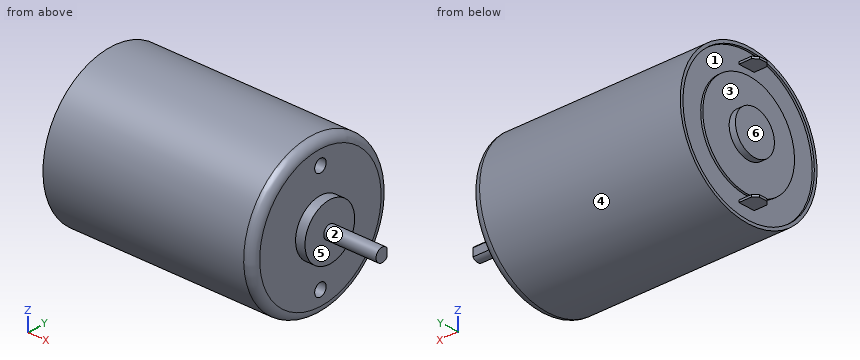
```python
from build123d import *

# Parameters (mm, degrees)
SKETCH1_R           = 17.9
MOTOR_BODY_DEPTH    = 25
SKETCH2_R           = 17.2
CUT_EXTRUDE1_DEPTH  = 0.5
SKETCH3_R           = 12
BOSS_EXTRUDE2_DEPTH = 0.5
SKETCH4_R           = 5.1
BOSS_EXTRUDE3_DEPTH = 1.5
FILLET1_R           = 2
SKETCH5_W           = 0.5
SKETCH5_H           = 4
BOSS_EXTRUDE4_DEPTH = 4
CHAMFER1_SIZE       = 1
SKETCH6_R           = 1.5
MOUNT_HOLES_DEPTH   = 6
SKETCH7_R           = 6.5
BOSS_EXTRUDE5_DEPTH = 2.25
SKETCH8_R           = 1.585
OUTPUT_SHAFT_DEPTH  = 12.5
CUT_EXTRUDE3_DEPTH  = 10


with BuildPart() as part:
    # Sketch1 → Motor-Body (new body, symmetric)
    with BuildSketch(Plane(origin=(0, 0, 0), x_dir=(0, 0, -1), z_dir=(1, 0, 0))):
        Circle(SKETCH1_R)
    extrude(amount=MOTOR_BODY_DEPTH, both=True)

    # Sketch2 → Cut-Extrude1 (cut)
    with BuildSketch(Plane.ZY.offset(25)):
        Circle(SKETCH2_R)
    extrude(amount=-CUT_EXTRUDE1_DEPTH, mode=Mode.SUBTRACT)

    # Sketch3 → Boss-Extrude2 (add, symmetric)
    with BuildSketch(Plane.ZY.offset(24.5)):
        Circle(SKETCH3_R)
    extrude(amount=BOSS_EXTRUDE2_DEPTH, both=True)

    # Sketch4 → Boss-Extrude3 (add, symmetric)
    with BuildSketch(Plane.ZY.offset(25)):
        Circle(SKETCH4_R)
    extrude(amount=BOSS_EXTRUDE3_DEPTH, both=True)

    # Fillet1
    fillet1_edges = [part.edges().sort_by_distance(p)[0] for p in [
        (25, 0, 17.9),
    ]]
    fillet(fillet1_edges, radius=FILLET1_R)

    # Sketch5 → Boss-Extrude4 (add)
    with BuildSketch(Plane.ZY.offset(24.5)):
        with Locations((-13.95, 0)):
            Rectangle(SKETCH5_W, SKETCH5_H)
        with Locations((13.95, 0)):
            Rectangle(SKETCH5_W, SKETCH5_H)
    extrude(amount=BOSS_EXTRUDE4_DEPTH)

    # Chamfer1
    chamfer1_edges = [part.edges().sort_by_distance(p)[0] for p in [
        (-28.5, 2, -13.95),
        (-28.5, -2, -13.95),
        (-28.5, 2, 13.95),
        (-28.5, -2, 13.95),
    ]]
    chamfer(chamfer1_edges, length=CHAMFER1_SIZE)

    # Sketch6 → Mount-Holes (cut)
    with BuildSketch(Plane(origin=(25, 0, 0), x_dir=(0, 0, -1), z_dir=(1, 0, 0))):
        with Locations((-12.5, 0)):
            Circle(SKETCH6_R)
        with Locations((12.5, 0)):
            Circle(SKETCH6_R)
    extrude(amount=-MOUNT_HOLES_DEPTH, mode=Mode.SUBTRACT)

    # Sketch7 → Boss-Extrude5 (add, symmetric)
    with BuildSketch(Plane(origin=(25, 0, 0), x_dir=(0, 0, -1), z_dir=(1, 0, 0))):
        Circle(SKETCH7_R)
    extrude(amount=BOSS_EXTRUDE5_DEPTH, both=True)

    # Sketch8 → Output-Shaft (add)
    with BuildSketch(Plane(origin=(27.25, 0, 0), x_dir=(0, 0, -1), z_dir=(1, 0, 0))):
        Circle(SKETCH8_R)
    extrude(amount=OUTPUT_SHAFT_DEPTH)

    # Sketch9 → Cut-Extrude3 (cut)
    with BuildSketch(Plane(origin=(39.75, 0, 0), x_dir=(0, 0, -1), z_dir=(1, 0, 0))):
        with BuildLine():
            Line((-0.927900857, 1.285), (0.927900857, 1.285))
            ThreePointArc((0.927900857, 1.285), (0, 1.585), (-0.927900857, 1.285))
        make_face()
    extrude(amount=-CUT_EXTRUDE3_DEPTH, mode=Mode.SUBTRACT)


solid = part.part
```
Check sheet for the modelled part. Datum: model origin and axes. Units: mm. Face numbers are marked on the shaded views. A direction names the side the tool comes from. Round coordinates to 2 decimals unless told otherwise and drop trailing zeros. Order: outer loops, then holes, each group sorted by start corner. A loop starts at its lowest first (then second) coordinate and runs counter-clockwise, first axis right, second up. Notation, with made-up numbers: (36, -32) - (77, -32) arc R23 ccw to (77, -24) - close; hole circle Ø8 at (62.25, 26.5). An arc over 180 degrees is marked (long way). Write item = value, one per line.
Q1. Thickness scan on line 1 along X through (y, z) = (14, 4.5); line 2 along X through (y, z) = (5, 2); line 3 along Y through (x, z) = (20, 12). Record the ranges inside material, lowest first.
Computed:
line_1 = -24.5 to 25
line_2 = -25 to 27.25
line_3 = -13.28 to -1.41, 1.41 to 13.28
Q2. Tool access check on the marked faces 4, 5 and 6. Record the directions out of +Z, -Z, +X, -X, +Y, -Y that give a thin tool (end or side, any length) a straight path to the whole face; none if there is none.
Computed:
face_4 = +X, -X
face_5 = +X
face_6 = -X, +Y, -Y
Q3. Draft check along Y on the marked faces 1, 2 and 3. Enter one of: pulls with the +Y half, pulls with the -Y half, needs draft (parallel to the pull), parting line crosses it, or undercut.
Computed:
face_1 = undercut
face_2 = parting line crosses it
face_3 = needs draft
Q4. Go/stop test with flat-tipped pins: pin 1 (17 mm diameter, centred on y = 7, z = -5.5, fed in from -X); pin 2 (3 mm diameter, centred on y = -13, z = 11, fed in from -X); pin 3 (2 mm diameter, centred on x = -27, y = -1, fed in from +Z); pin 4 (3 mm diameter, centred on x = 30.5, y = -7, fed in from -Z). Record where each tip stops, or that it passes through.
Computed:
pin_1 = -26.5
pin_2 = -25
pin_3 = 14.2
pin_4 = through
Q5. Section check A-A (z = 0). Record the boundary of the cut face in (x, y) (3 decimals).
Computed:
outline = (-26.5, -5.1) - (-25, -5.1) - (-25, -12) - (-24.5, -12) - (-24.5, -17.2) - (-25, -17.2) - (-25, -17.9) - (23, -17.9) arc R2 ccw to (25, -15.9) - (25, -6.5) - (27.25, -6.5) - (27.25, -1.585) - (39.75, -1.585) - (39.75, 1.285) - (29.75, 1.285) - (29.75, 1.585) - (27.25, 1.585) - (27.25, 6.5) - (25, 6.5) - (25, 15.9) arc R2 ccw to (23, 17.9) - (-25, 17.9) - (-25, 17.2) - (-24.5, 17.2) - (-24.5, 12) - (-25, 12) - (-25, 5.1) - (-26.5, 5.1) - close
Q6. Section check B-B (x = 8.5). Record the boundary of the cut face in (y, z).
Computed:
outline = circle Ø35.8 at (0, 0)
